Work out the finished part from the listing and answer in its coordinate system (mm). A direction names the side the tool comes from. Round coordinates to 2 decimals unless told otherwise and drop trailing zeros. Write each loop counter-clockwise with the first axis right and the second up, starting at its lowest first coordinate (ties: lowest second). Pieces come first, ordered by that corner, then holes.
from build123d import *

# Parameters (mm, degrees)
BOSS_EXTRUDE1_DEPTH = 3
FILLET1_R           = 20


with BuildPart() as part:
    # Sketch1 → Boss-Extrude1 (new body)
    with BuildSketch(Plane.XY):
        with BuildLine():
            Line((-0.5, -84.19), (0.5, -84.19))
            Line((0.5, -84.19), (25, -84.19))
            ThreePointArc((25, -84.19), (60.355339059, -69.545339059), (75, -34.19))
            Line((75, -34.19), (75, 63.81))
            ThreePointArc((75, 63.81), (71.192388155, 73.002388155), (62, 76.81))
            Line((62, 76.81), (-62, 76.81))
            ThreePointArc((-62, 76.81), (-71.192388155, 73.002388155), (-75, 63.81))
            Line((-75, 63.81), (-75, -34.19))
            ThreePointArc((-75, -34.19), (-60.355339059, -69.545339059), (-25, -84.19))
            Line((-25, -84.19), (-0.5, -84.19))
        make_face()
        with BuildLine():
            Line((50, 51.81), (-50, 51.81))
            Line((-50, 51.81), (-50, -34.19))
            ThreePointArc((-50, -34.19), (-42.67766953, -51.86766953), (-25, -59.19))
            Line((-25, -59.19), (-0.5, -59.19))
            Line((-0.5, -59.19), (0.5, -59.19))
            Line((0.5, -59.19), (25, -59.19))
            ThreePointArc((25, -59.19), (42.67766953, -51.86766953), (50, -34.19))
            Line((50, -34.19), (50, 51.81))
        make_face(mode=Mode.SUBTRACT)
    extrude(amount=BOSS_EXTRUDE1_DEPTH)

    # Fillet1
    fillet1_edges = [part.edges().sort_by_distance(p)[0] for p in [
        (50, 51.81, 1.5),
        (-50, 51.81, 1.5),
    ]]
    fillet(fillet1_edges, radius=FILLET1_R)


solid = part.part
Q1. Find section A-A (y = -14.5). Determine the outline of the cut face in (x, z), plus the area to 3 significant figures.
Q2. A tool of negligible diameter and unlimited length cuts with its end or side. For faces 1 (the face through (43.986, 46.107, 1.521)), 2 (the face through (-51, -3, 3)), from which of +Z, -Z, +X, -X, +Y, -Y can it reach the whole face along a straight path? Write none if from no direction.
Q3. Find section B-B (x = 23). Determine the outline of the cut face in (y, z).
Q4. The mould has two halves that part along Y. Classify faces 3 (the face through (-71.091, 73.103, 1.479)), 4 (the face through (-60.7, -69.2, 1.5)), 5 (the face through (-43.986, 46.107, 1.521)), 6 (the face through (42.482, -52.061, 1.479)): +Y half, -Y half, draft (parallel to the pull), parting line (faces both ways), or undercut.
Q5. Find the intervals of material crossed by L1, parallel to X at y = 29, z = 2.8; L2, parallel to Y at x = 11.5, z = 1.7; L3, parallel to Y at x = -27.5, z = 1.95, in increasing order.
Q6. Find section C-C (z = 0.55). Determine the outline of the cut face in (x, y), plus the area to 3 significant figures.
Q7. Find section D-D (x = 57.5). Determine the outline of the cut face in (y, z).
Report:
1. outline: (-75, 0) - (-50, 0) - (-50, 3) - (-75, 3) - close; (50, 0) - (75, 0) - (75, 3) - (50, 3) - close
1. area: 150 mm2
2. face 1: +Z, -Z
2. face 2: +Z, +X, -X, +Y, -Y
3. outline: (-84.19, 0) - (-59.19, 0) - (-59.19, 3) - (-84.19, 3) - close; (51.81, 0) - (76.81, 0) - (76.81, 3) - (51.81, 3) - close
4. face 3: +Y half
4. face 4: -Y half
4. face 5: undercut
4. face 6: undercut
5. L1: x = -75 to -50, 50 to 75
5. L2: y = -84.19 to -59.19, 51.81 to 76.81
5. L3: y = -84.13 to -59.06, 51.81 to 76.81
6. outline: (-75, -34.19) arc R50 ccw to (-25, -84.19) - (25, -84.19) arc R50 ccw to (75, -34.19) - (75, 63.81) arc R13 ccw to (62, 76.81) - (-62, 76.81) arc R13 ccw to (-75, 63.81) - close; hole (-50, -34.19) arc R25 ccw to (-25, -59.19) - (25, -59.19) arc R25 ccw to (50, -34.19) - (50, 31.81) arc R20 ccw to (30, 51.81) - (-30, 51.81) arc R20 ccw to (-50, 31.81) - close
6. area: 12,300 mm2
7. outline: (-72.19, 0) - (76.81, 0) - (76.81, 3) - (-72.19, 3) - close
